Study the drawing (mm; zero at the part's minimum x, y, z) and answer. A direction names the side the tool comes from. Give positions to 0.01 mm unless a question says otherwise; leave off trailing zeros.
Item 1: Find the intervals of material crossed by line 1 along Z through (x, y) = (1.5, 3) (1 decimal); line 2 along Y through (x, z) = (3.5, 35) (1 decimal), in increasing order.
Item 2: Which of the six approach directions +Z, -Z, +X, -X, +Y, -Y give full straight-line access (tool end or side, diameter ignored) to the marked faces 1 and 2?
Item 3: Given pin 1 Ø2 at (y, z) = (1, 29.5) entering from +X; pin 2 Ø1 at (y, z) = (4.5, 37) entering from -X; pin 3 Ø1.5 at (x, z) = (6.5, 36) entering from +Y, each flat-ended and moving along its own axis, determine where each tip first touches the part or whether it passes through.
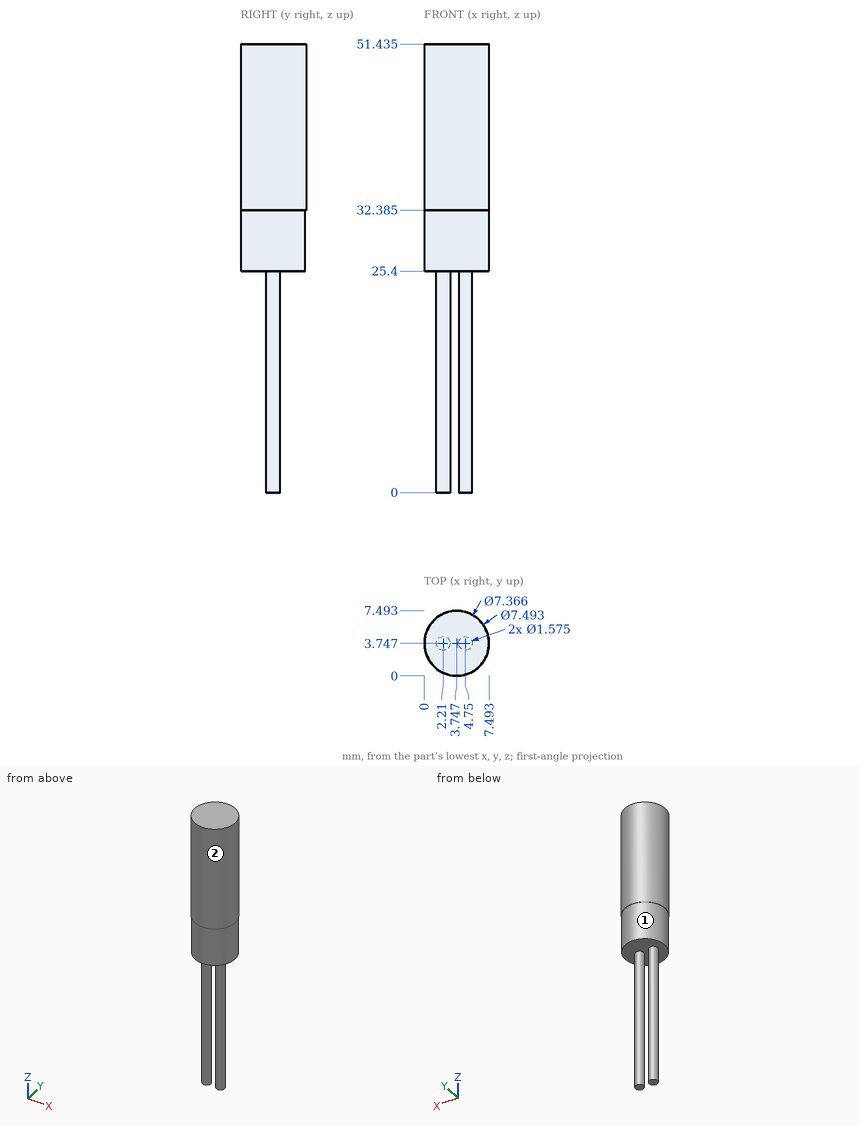
Response values:
1. line 1: z = 25.4 to 51.4
1. line 2: y = 0 to 7.5
2. face 1: -Z
2. face 2: +Z, -Z
3. pin 1: stops at x = 6.99
3. pin 2: stops at x = 0.01
3. pin 3: stops at y = 6.91
